Build history of the part. All positions in model axes, mm. Face numbers are marked on the shaded views. A direction names the side the tool comes from. Give positions to 0.01 mm unless a question says otherwise; leave off trailing zeros. Loops run counter-clockwise (first coordinate to the right, second up) from the corner with the lowest first, then second, coordinate; pieces in that order, holes last. Notation, with made-up numbers: M 32,35.25 L 75,35.25 A13 ccw 75,40.25 Z; hole C 20.25,50 d2. An arc over 180 degrees is marked long. Put each result on its own line as item: value.
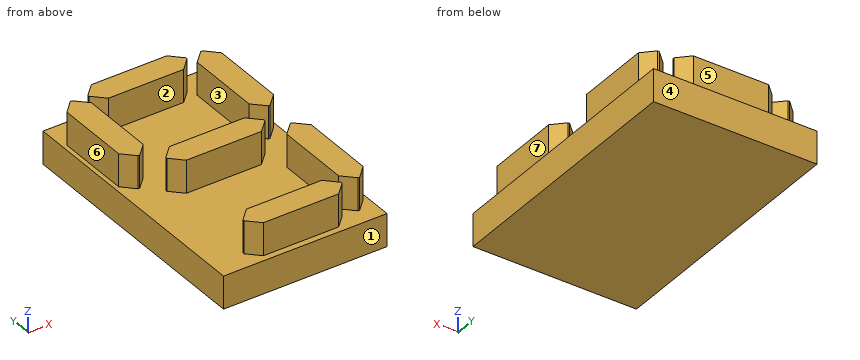
```python
from build123d import *

# Parameters (mm, degrees)
F0_W     = 10
F0_H     = 16
F1_DEPTH = 2
F2_W     = 1.5
F2_H     = 6
F2_W_2   = 6
F2_H_2   = 1.5
F3_DEPTH = 2
F4_SIZE  = 0.7


# Not quite as in the source:
# - a feature names something its author has since deleted; it is built from what else it names


with BuildPart() as f1:
    # F0 (on Top) → F1 (new body)
    with BuildSketch(Plane.XY):
        Rectangle(F0_W, F0_H)
    extrude(amount=-F1_DEPTH)

    # F2 (on face) → F3 (join)
    with BuildSketch(Plane.XY):
        with Locations((-3.9874258153, 3.9691079506)):
            Rectangle(F2_W, F2_H)
        with Locations((0, 6.8687610328)):
            Rectangle(F2_W_2, F2_H_2)
        with Locations((3.9874258153, 3.9691079506)):
            Rectangle(F2_W, F2_H)
        with Locations((0.0284713751, 0.0055548735)):
            Rectangle(F2_W_2, F2_H_2)
        with Locations((0, -6.8687610328)):
            Rectangle(F2_W_2, F2_H_2)
        with Locations((3.9874258153, -3.9691079506)):
            Rectangle(F2_W, F2_H)
    extrude(amount=F3_DEPTH)

    # F4
    f4_edges = [f1.edges().sort_by_distance(p)[0] for p in [
        (3, 6.118761, 1),
        (3.237426, 6.969108, 1),
        (3.237426, 0.969108, 1),
        (4.737426, 0.969108, 1),
        (3.237426, -0.969108, 1),
        (3.028471, -0.744445, 1),
        (-2.971529, -0.744445, 1),
        (-2.971529, 0.755555, 1),
        (-3.237426, 0.969108, 1),
        (-4.737426, 0.969108, 1),
        (-4.737426, 6.969108, 1),
        (-3, 6.118761, 1),
        (-3, 7.618761, 1),
        (3.237426, -6.969108, 1),
        (4.737426, -6.969108, 1),
        (3, -7.618761, 1),
        (-3, -7.618761, 1),
        (-3, -6.118761, 1),
        (3.028471, 0.755555, 1),
        (4.737426, -0.969108, 1),
        (3, -6.118761, 1),
        (4.737426, 6.969108, 1),
        (3, 7.618761, 1),
        (-3.237426, 6.969108, 1),
    ]]
    chamfer(f4_edges, length=F4_SIZE)


solid = f1.part
```
Q1. Slice it at C-C (z = 1). State how many separate pieces and enclosed holes the cut face has, and give its area (3 significant figures).
Here are the results:
separate pieces: 6
enclosed holes: 0
area: 48.1 mm²
Q2. Drop flat-ended pins along their axis: pin 1 Ø0.6 at (x, z) = (0.5, 1.5) entering from -Y; pin 2 Ø1 at (y, z) = (4.5, 1.5) entering from +X; pin 3 Ø4 at (x, y) = (-1.5, -3.5) entering from +Z. Give the stop position or say it passes through.
Here are the results:
pin 1: y = -7.62
pin 2: x = 4.74
pin 3: z = 0
Q3. Slice it at D-D (y = 5.5). List the corners of the cut face in (x, z).
Here are the results:
outline: M -5,-2 L 5,-2 L 5,0 L 4.74,0 L 4.74,2 L 3.24,2 L 3.24,0 L -3.24,0 L -3.24,2 L -4.74,2 L -4.74,0 L -5,0 Z
Q4. Mould opens along Y. For the marked faces 1, 2, 3 and 4 say: pulls with the +Y half, pulls with the -Y half, needs draft (parallel to the pull), parting line crosses it, or undercut.
Here are the results:
face 1: pulls with the -Y half
face 2: undercut
face 3: needs draft
face 4: pulls with the +Y half
Q5. Slice it at A-A (y = -4.75). List the corners of the cut face in (x, z), and give its area (3 significant figures).
Here are the results:
outline: M -5,-2 L 5,-2 L 5,0 L 4.74,0 L 4.74,2 L 3.24,2 L 3.24,0 L -5,0 Z
area: 23.0 mm²
Q6. Tool access for the marked faces 5, 6 and 7: list every direction of +Z, -Z, +X, -X, +Y, -Y with a clear straight run to the whole face (end or side of a thin tool).
Here are the results:
face 5: +Z, +X, -X, +Y
face 6: +Z, -X, +Y, -Y
face 7: +Z, +X, +Y, -Y
Q7. Slice it at B-B (x = 0.75). List the corners of the cut face in (y, z), and give its area (3 significant figures).
Here are the results:
outline: M -8,-2 L 8,-2 L 8,0 L 7.62,0 L 7.62,2 L 6.12,2 L 6.12,0 L 0.76,0 L 0.76,2 L -0.74,2 L -0.74,0 L -6.12,0 L -6.12,2 L -7.62,2 L -7.62,0 L -8,0 Z
area: 41.0 mm²
Q8. Probe line 1 (Y direction, x = 0.75, z = 1.75); line 2 (X direction, y = 6, z = 0.7); line 3 (X direction, y = -1.75, z = 1). List the from-to ranges inside material, lowest first. Write a range as from..to.
Here are the results:
line 1: -7.62..-6.12, -0.74..0.76, 6.12..7.62
line 2: -4.74..-3.24, 3.24..4.74
line 3: 3.24..4.74
